from build123d import *

# Parameters (mm, degrees)
BOSS_EXTRUDE1_DEPTH = 7.5
SKETCH2_R           = 5
SKETCH2_R_2         = 2
CUT_EXTRUDE1_DEPTH  = 171.403198327
SKETCH3_R           = 9
BOSS_EXTRUDE2_DEPTH = 7.5
SKETCH4_R           = 5
CUT_EXTRUDE2_DEPTH  = 171.403198327


with BuildPart() as part:
    # Sketch1 → Boss-Extrude1 (new body)
    with BuildSketch(Plane(origin=(0, 0, 0), x_dir=(1, 0, 0), z_dir=(0, 1, 0))):
        with BuildLine():
            Line((0, 9), (170, 9))
            Line((170, 9), (170, -9))
            Line((170, -9), (0, -9))
            ThreePointArc((0, -9), (-9, 0), (0, 9))
        make_face()
    extrude(amount=BOSS_EXTRUDE1_DEPTH)

    # Sketch2 → Cut-Extrude1 (cut, through all)
    with BuildSketch(Plane(origin=(0, 7.5, 0), x_dir=(1, 0, 0), z_dir=(0, 1, 0))):
        with Locations(Location((0, 0, 0), (0, 0, 270))):
            Circle(SKETCH2_R)
        with Locations(Location((160, 0, 0), (0, 0, 270))):
            Circle(SKETCH2_R_2)
        with Locations(Location((140, 0, 0), (0, 0, 270))):
            Circle(SKETCH2_R_2)
    extrude(amount=-CUT_EXTRUDE1_DEPTH, mode=Mode.SUBTRACT)

    # Sketch3 → Boss-Extrude2 (add)
    with BuildSketch(Plane(origin=(0, 7.5, 0), x_dir=(1, 0, 0), z_dir=(0, 1, 0))):
        with Locations(Location((0, 0, 0), (0, 0, 270))):
            Circle(SKETCH3_R)
    extrude(amount=BOSS_EXTRUDE2_DEPTH)

    # Sketch4 → Cut-Extrude2 (cut, through all)
    with BuildSketch(Plane.XZ.offset(-7.5)):
        with Locations(Location((0, 0, 0), (0, 0, 90))):
            Circle(SKETCH4_R)
    extrude(amount=-CUT_EXTRUDE2_DEPTH, mode=Mode.SUBTRACT)


solid = part.part
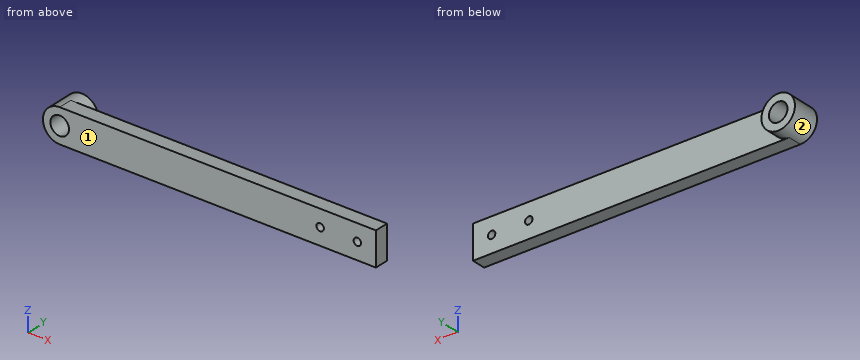
Design review of the part built by this model. Coordinates are the model's own, in mm. Face numbers are marked on the shaded views. A direction names the side the tool comes from. Coordinates: 2 decimals unless noted, no trailing zeros. Loops run counter-clockwise (first coordinate to the right, second up) from the corner with the lowest first, then second, coordinate; pieces in that order, holes last. Notation, with made-up numbers: (-3, 8.5) - (21, 8.5) arc R36 ccw to (21, 44.5) - close; hole circle Ø9 at (34, 65). An arc over 180 degrees is marked (long way). Use CSV: the item, a comma, the result in double quotes. Start each with the question number.
1. Add section B-B on x = 140. Give the boundary of the cut face in (y, z).
2. To check wall thickness, follow probe 1 along X at (y, z) = (6.25, 0); probe 2 along X at (y, z) = (11.25, 0); probe 3 along Z at (x, y) = (140, 2.75). State the ranges of each line that lie inside material, in increasing order.
3. For the marked faces 1 and 2, list the 3-axis set-ups (+Z, -Z, +X, -X, +Y, -Y) from which the entire face can be reached by the end or side of a thin tool; tool diameter is ignored.
4. Clearance check with flat-ended pins moving along their axes: pin 1 (6 mm diameter, centred on x = 34.5, z = 0, fed in from -Y); pin 2 (5 mm diameter, centred on x = 160, z = 0, fed in from +Y); pin 3 (1.5 mm diameter, centred on y = 7.5, z = 4.5, fed in from -X). State where each tip first meets the part, or that it passes through.
5. Add section D-D on y = 13. Give the boundary of the cut face in (x, z).
6. Add section C-C on y = 5. Give the boundary of the cut face in (x, z), plus the area to 3 significant figures.
7. Add section A-A on z = 0. Give the boundary of the cut face in (x, y).
Resolved:
1,outline,"(0, -9) - (7.5, -9) - (7.5, -2) - (0, -2) - close; (0, 2) - (7.5, 2) - (7.5, 9) - (0, 9) - close"
2,probe 1,"-9 to -5, 5 to 138, 142 to 158, 162 to 170"
2,probe 2,"-9 to -5, 5 to 9"
2,probe 3,"-9 to -2, 2 to 9"
3,face 1,"+Z, -Z, +X, -X, -Y"
3,face 2,"+Y"
4,pin 1,"y = 0"
4,pin 2,"y = 7.5"
4,pin 3,"x = -8.18"
5,outline,"circle Ø18 at (0, 0); hole circle Ø10 at (0, 0)"
6,outline,"(0, -9) - (170, -9) - (170, 9) - (0, 9) arc R9 ccw to start; hole circle Ø10 at (0, 0); hole circle Ø4 at (140, 0); hole circle Ø4 at (160, 0)"
6,area,"3,080 mm2"
7,outline,"(-9, 0) - (-5, 0) - (-5, 15) - (-9, 15) - close; (5, 0) - (138, 0) - (138, 7.5) - (9, 7.5) - (9, 15) - (5, 15) - close; (142, 0) - (158, 0) - (158, 7.5) - (142, 7.5) - close; (162, 0) - (170, 0) - (170, 7.5) - (162, 7.5) - close"
